```python
from build123d import *

# Parameters (mm, degrees)
EXTRUDE1_DEPTH           = 4
EXTRUDE1_DEPTH_BACK      = 4
SKETCH2_W                = 3.8
SKETCH2_H                = 12
SKETCH2_W_2              = 21
SKETCH2_H_2              = 3.8
EXTRUDE2_DEPTH           = 3
CHAMFER1_SIZE            = 3
CHAMFER1_OF_MIRROR1_SIZE = 3
CHAMFER2_SIZE            = 1.4
EXTRUDE3_REACH           = 30.24
SKETCH4_R                = 3
FILLET1_R                = 0.8
EXTRUDE4_REACH           = 30.24
SKETCH5_R                = 3
FILLET2_R                = 1


with BuildPart() as part:
    # Sketch1 → Extrude1 (new, two sides: drawn at the far end of the back side and taken through both)
    with BuildSketch(Plane.XY.offset(-EXTRUDE1_DEPTH_BACK)):
        Polygon((0, 0), (0, 14.5), (-6.5, 14.5), (-6.5, -6.5), (23.2, -6.5), (23.2, 0), align=None)
    extrude(amount=EXTRUDE1_DEPTH + EXTRUDE1_DEPTH_BACK)

    # Sketch2 → Extrude2 (add)
    with BuildSketch(Plane.XY.offset(4)):
        with Locations((-3.2, 8.5)):
            Rectangle(SKETCH2_W, SKETCH2_H)
        with Locations((12.7, -3.2)):
            Rectangle(SKETCH2_W_2, SKETCH2_H_2)
    extrude2 = extrude(amount=EXTRUDE2_DEPTH)

    # Chamfer1
    chamfer1_edges = [part.edges().sort_by_distance(p)[0] for p in [
        (23.2, -3.2, 7),
    ]]
    chamfer(chamfer1_edges, length=CHAMFER1_SIZE)

    # Mirror1: Extrude2 across plane
    add(extrude2.mirror(Plane.XY))

    # Chamfer1 of Mirror1
    chamfer1_of_mirror1_edges = [part.edges().sort_by_distance(p)[0] for p in [
        (23.2, -3.2, -7),
    ]]
    chamfer(chamfer1_of_mirror1_edges, length=CHAMFER1_OF_MIRROR1_SIZE)

    # Chamfer2
    # the kernel refuses this chamfer: 1.4 mm, written as the material it takes off along each edge
    with BuildSketch(Plane(origin=(23.2, 0, 7.600356183), x_dir=(0.027495876610586112, -0.9996219169112968, 0), z_dir=(0, 0, -1))) as chamfer2_piece_1:
        Polygon((CHAMFER2_SIZE * 0.999621916911, CHAMFER2_SIZE * 0.0274958766106), (-CHAMFER2_SIZE * 0.0274958766106, CHAMFER2_SIZE * 0.999621916911), (0, 0), align=None)
    extrude(amount=15.200712366, mode=Mode.SUBTRACT)
    with BuildSketch(Plane(origin=(23.2, -6.5, 7.600356183), x_dir=(0.02749587661058614, 0.9996219169112968, 0), z_dir=(0, 0, -1))) as chamfer2_piece_2:
        Polygon((CHAMFER2_SIZE * 0.999621916911, -CHAMFER2_SIZE * 0.0274958766106), (-CHAMFER2_SIZE * 0.0274958766106, -CHAMFER2_SIZE * 0.999621916911), (0, 0), align=None)
    extrude(amount=15.200712366, mode=Mode.SUBTRACT)

    # Sketch4 → Extrude3 (cut, up to next)
    with BuildSketch(Plane(origin=(0, 0, 0), x_dir=(1, 0, 0), z_dir=(0, 1, 0)), mode=Mode.PRIVATE) as extrude3_sk1:
        with Locations(Location((14.5, 0, 0), (0, 0, 270))):
            Circle(SKETCH4_R)
    extrude3_tool1 = extrude(extrude3_sk1.sketch, amount=-EXTRUDE3_REACH, mode=Mode.PRIVATE) & part.part
    add(extrude3_tool1.solids().sort_by_distance((14.5, 0, 0))[0], mode=Mode.SUBTRACT)

    # Fillet1
    fillet1_edges = [part.edges().sort_by_distance(p)[0] for p in [
        (-6.5, 14.5, 0),
        (0, 14.5, 0),
    ]]
    fillet(fillet1_edges, radius=FILLET1_R)

    # Sketch5 → Extrude4 (cut, up to next)
    with BuildSketch(Plane(origin=(0, 0, 0), x_dir=(0, 0, -1), z_dir=(1, 0, 0)), mode=Mode.PRIVATE) as extrude4_sk1:
        with Locations(Location((0, 7.6, 0), (0, 0, 90))):
            Circle(SKETCH5_R)
    extrude4_tool1 = extrude(extrude4_sk1.sketch, amount=-EXTRUDE4_REACH, mode=Mode.PRIVATE) & part.part
    add(extrude4_tool1.solids().sort_by_distance((0, 7.6, 0))[0], mode=Mode.SUBTRACT)

    # Fillet2
    fillet2_edges = [part.edges().sort_by_distance(p)[0] for p in [
        (0, 0, 0),
    ]]
    fillet(fillet2_edges, radius=FILLET2_R)


solid = part.part
```
Work out the finished part from the listing and answer in its coordinate system (mm). A direction names the side the tool comes from. Coordinates: 2 decimals unless noted, no trailing zeros. Write each loop counter-clockwise with the first axis right and the second up, starting at its lowest first coordinate (ties: lowest second). Pieces come first, ordered by that corner, then holes.
Q1. Find the intervals of material crossed by line 1 (Z direction, x = -4.75, y = 7.6); line 2 (X direction, y = 11, z = 4.5); line 3 (Z direction, x = -1.25, y = -4), in increasing order.
Q2. Determine the mould class of faces 1 (the face through (-3.2, 4.6, 0.1)), 2 (the face through (-6.5, 4, 0)), 3 (the face through (13, -1.3, -5)) for opening direction Y: released by +Y, released by -Y, zero draft, split by the parting line, or undercut.
Q3. A cutting plane is placed at B-B, the plane y = 7.6. Give the vertices of the cut face in (x, z).
Q4. Each of these flat-tipped pins is pushed along its axis until it touches: pin 1 Ø12 at (x, y) = (13, 0) entering from +Z; pin 2 Ø0.9 at (y, z) = (9.5, -5.5) entering from +X; pin 3 Ø7 at (y, z) = (7.6, 0) entering from +X; pin 4 Ø1.5 at (x, z) = (9, -5.5) entering from +Y. Where does it stop, or does it pass through?
Q5. A cutting plane is placed at C-C, the plane z = -4.5. Give the vertices of the cut face in (x, y), then the cut area to 4 significant figures.
Q6. A cutting plane is placed at A-A, the plane z = 0. Give the vertices of the cut face in (x, y).
Q7. Which of the six approach directions +Z, -Z, +X, -X, +Y, -Y give full straight-line access (tool end or side, diameter ignored) to faces 4 (the face through (-1.3, 8, -5)), 5 (the face through (13, -5.1, -5)), 6 (the face through (0, 4, 0)), 7 (the face through (-5.1, 8, -5))?
Findings below:
1. line 1: z = -7 to -3, 3 to 7
1. line 2: x = -5.1 to -1.3
1. line 3: z = -4 to 4
2. face 1: undercut
2. face 2: zero draft
2. face 3: released by +Y
3. outline: (-6.5, -4) - (-5.1, -4) - (-5.1, -7) - (-1.3, -7) - (-1.3, -4) - (0, -4) - (0, -3) - (-6.5, -3) - close; (-6.5, 3) - (0, 3) - (0, 4) - (-1.3, 4) - (-1.3, 7) - (-5.1, 7) - (-5.1, 4) - (-6.5, 4) - close
4. pin 1: stops at z = 7
4. pin 2: stops at x = -1.3
4. pin 3: stops at x = 0
4. pin 4: stops at y = -1.3
5. outline: (-5.1, 2.5) - (-1.3, 2.5) - (-1.3, 14.5) - (-5.1, 14.5) - close; (2.2, -5.1) - (22.7, -5.1) - (22.7, -1.3) - (2.2, -1.3) - close
5. area: 123.5 mm2
6. outline: (-6.5, -6.5) - (11.5, -6.5) - (11.5, 0) - (1, 0) arc R1 cw to (0, 1) - (0, 4.6) - (-6.5, 4.6) - close; (-6.5, 10.6) - (0, 10.6) - (0, 13.7) arc R0.8 ccw to (-0.8, 14.5) - (-5.7, 14.5) arc R0.8 ccw to (-6.5, 13.7) - close; (17.5, -6.5) - (21.8, -6.5) - (23.2, -5.1) - (23.2, -1.4) - (21.8, 0) - (17.5, 0) - close
7. face 4: -Z, +X, +Y, -Y
7. face 5: -Z, +X, -X, -Y
7. face 6: +Z, -Z, +X, +Y
7. face 7: -Z, -X, +Y, -Y
